Can you work these out from the model? Positions are in its coordinate system, mm. Face numbers are marked on the shaded views. A direction names the side the tool comes from. Give positions to 0.01 mm unless a question says otherwise; leave off trailing zeros. Order: outer loops, then holes, each group sorted by start corner. A loop starts at its lowest first (then second) coordinate and runs counter-clockwise, first axis right, second up. Notation, with made-up numbers: (49.5, 4.25) - (94.5, 4.25) arc R26 cw to (94.5, 41.25) - close; hole circle Ø1 at (-8, -32.75). An arc over 180 degrees is marked (long way). Return JSON: item names as keys, results as strings.
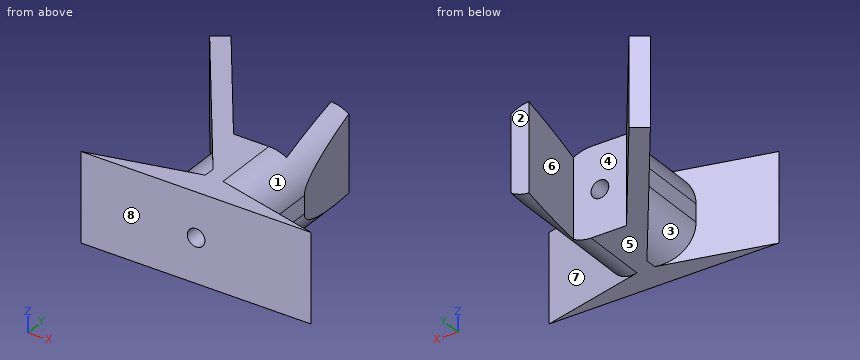
```python
from build123d import *

# Parameters (mm, degrees)
BOSS_EXTRUDE1_DEPTH     = 12.7
FILLET2_R               = 5.08
SKETCH5_R               = 1.27
CUT_EXTRUDE1_DEPTH      = 1
CUT_EXTRUDE1_DEPTH_BACK = 32.936884148


with BuildPart() as part:
    # Sketch2 → Boss-Extrude1 (new body)
    with BuildSketch(Plane.XY):
        Polygon((-10.16, 13.500858924), (-2.54, 13.500858924), (-4.779352655, 26.200858924), (-2.239352655, 26.200858924), (0, 13.500858924), (0, 2.54), (10.16, 0), (0, 0), (-12.7, 0), (-22.86, 0), (-12.7, 2.54), (-12.7, 12.7), (-25.149690029, 30.48), (-23.069043837, 31.936884148), align=None)
    extrude(amount=BOSS_EXTRUDE1_DEPTH)

    # Fillet2
    fillet2_edges = [part.edges().sort_by_distance(p)[0] for p in [
        (-12.7, 7.62, 12.7),
        (-12.7, 7.62, 0),
        (0, 8.020429462, 0),
        (0, 8.020429462, 12.7),
    ]]
    fillet(fillet2_edges, radius=FILLET2_R)

    # Sketch5 → Cut-Extrude1 (cut, two sides)
    with BuildSketch(Plane.XZ) as cut_extrude1_sk:
        with Locations((-6.35, 6.35)):
            Circle(SKETCH5_R)
    extrude(amount=CUT_EXTRUDE1_DEPTH, mode=Mode.SUBTRACT)
    extrude(cut_extrude1_sk.sketch, amount=-CUT_EXTRUDE1_DEPTH_BACK, mode=Mode.SUBTRACT)


solid = part.part
```
1. On a 3-axis mill with a long thin cutter (end or side, diameter ignored), from which of +Z, -Z, +X, -X, +Y, -Y can I reach the whole of each face in a straight line? I mean the marked faces 1, 2, 3, 4 and 5. Say none if no direction works.
Checks:
{"face 1": "+Z, +X, +Y", "face 2": "+Z, -Z, +X, +Y", "face 3": "-Z, -X", "face 4": "+Z, -Z", "face 5": "-Z, +X, -X, +Y, -Y"}
2. Suppose I cut it at C-C (y = 20.5). List the corners of the cut face in (x, z) for me, plus the area to 3 significant figures.
Checks:
{"outline": "(-18.16, 0) - (-15.06, 0) - (-15.06, 12.7) - (-18.16, 12.7) - close; (-3.77, 0.17) arc R5.08 ccw to (-1.23, 1.76) - (-1.23, 10.94) arc R5.08 ccw to (-3.77, 12.53) - close", "area": "67.6 mm^2"}
3. Thinking about a two-plate mould opening in Y: for the marked faces 6, 7 and 8, which applies, +Y half, -Y half, draft (parallel to the pull), parting line (faces both ways), or undercut?
Checks:
{"face 6": "undercut", "face 7": "+Y half", "face 8": "-Y half"}
4. Suppose I cut it at A-A (x = -6.35). List the corners of the cut face in (y, z) for me, plus the area to 3 significant figures.
Checks:
{"outline": "(0, 0) - (13.5, 0) - (13.5, 5.08) - (0, 5.08) - close; (0, 7.62) - (13.5, 7.62) - (13.5, 12.7) - (0, 12.7) - close", "area": "137 mm^2"}
5. For pin 1 Ø6 at (y, z) = (10, 10) entering from +X; pin 2 Ø1 at (y, z) = (12.5, 9.5) entering from -X; pin 3 Ø6 at (x, y) = (-19, 5) entering from +Z; pin 4 Ø1.3 at (y, z) = (10, 6) entering from -X, each with a flat end and sliding along its axis, tell me the tip position at first contact or that it passes through.
Checks:
{"pin 1": "x = 0", "pin 2": "x = -12.91", "pin 3": "through", "pin 4": "x = -12.7"}
6. Suppose I cut it at B-B (z = 6.35). List the corners of the cut face in (x, y) for me.
Checks:
{"outline": "(-25.15, 30.48) - (-12.7, 12.7) - (-12.7, 2.54) - (-22.86, 0) - (-7.62, 0) - (-7.62, 13.5) - (-10.16, 13.5) - (-23.07, 31.94) - close; (-5.08, 0) - (10.16, 0) - (0, 2.54) - (0, 13.5) - (-2.24, 26.2) - (-4.78, 26.2) - (-2.54, 13.5) - (-5.08, 13.5) - close"}
7. Suppose I cut it at D-D (y = 8.5). List the corners of the cut face in (x, z) for me.
Checks:
{"outline": "(-12.7, 5.08) arc R5.08 ccw to (-9.76, 0.47) - (-9.76, 0) - (-5.08, 0) arc R5.08 ccw to (0, 5.08) - (0, 7.62) arc R5.08 ccw to (-5.08, 12.7) - (-9.76, 12.7) - (-9.76, 12.23) arc R5.08 ccw to (-12.7, 7.62) - close; hole circle Ø2.54 at (-6.35, 6.35)"}
8. If I drill on L1, parallel to Z at x = -6.35, y = 4.25; L2, parallel to Y at x = -10, z = 4; L3, parallel to X at y = 16, z = 3, over which ranges is the centre line in solid material (lowest first)? Write a range as [from, to].
Checks:
{"L1": "[0, 5.08], [7.62, 12.7]", "L2": "[0, 13.5]", "L3": "[-15.01, -11.91], [-2.98, -0.45]"}
